Here's how the part is built. I have some questions about the finished solid (model axes, mm). A direction names the side the tool comes from. Coordinates: 2 decimals unless noted, no trailing zeros. Write each loop counter-clockwise with the first axis right and the second up, starting at its lowest first coordinate (ties: lowest second). Pieces come first, ordered by that corner, then holes.
(1) Imagine slicing it at A-A, the plane x = 0. List the corners of the cut face in (y, z) for me.
(2) Thinking about a two-plate mould opening in X: for faces 4 (the flat face through (-40, 0, 6)), 5 (the cylindrical face through (20.765, -39.923, -1.479)), 6 (the cylindrical face through (-3, 0, 0)), which applies, released by +X, released by -X, zero draft, split by the parting line, or undercut?
(3) Imagine slicing it at D-D, the plane x = -10. List the corners of the cut face in (y, z) for me, plus the area to 3 significant figures.
(4) Please list where these lines run through material, in increasing order: probe 1 along Y at (x, z) = (0, -2.5); probe 2 along Y at (x, z) = (18, 2); probe 3 along Y at (x, z) = (0, 1).
(5) Imagine slicing it at C-C, the plane z = 1.5. State how many separate pieces and enclosed holes the cut face has, plus the area to 3 significant figures.
(6) For pin 1 Ø5.5 at (x, y) = (0, 0) entering from -Z; pin 2 Ø4 at (x, y) = (-11.5, -0.5) entering from -Z; pin 3 Ø13 at (x, y) = (2, -1) entering from +Z; pin 4 Ø5 at (y, z) = (-34, -2) entering from +X, each with a flat end and sliding along its axis, tell me the tip position at first contact or that it passes through.
(7) Which directions (+Z, -Z, +X, -X, +Y, -Y) give clear straight access to the entire face, cutting with the end or side of a thin tool? Please do faces 1 (the flat face through (-3, -1, 4)), 2 (the flat face through (20, 0, 6)), 3 (the cylindrical face through (22.997, -34.773, 2.958)).
```python
from build123d import *

# Parameters (mm, degrees)
SKETCH_1_R           = 45
EXTRUDE_1_DEPTH      = 3
SKETCH_2_R           = 3
EXTRUDE_2_DEPTH      = 6
EXTRUDE_3_DEPTH      = 4
EXTRUDE_3_DEPTH_BACK = 5
SKETCH_3_R           = 6
CUT_EXTRUDE_1_REACH  = 66.273
SKETCH_4_R           = 3
SKETCH_5_R           = 3
EXTRUDE_4_DEPTH      = 6


with BuildPart() as part:
    # 草图1 → 凸台-拉伸1 (new body)
    with BuildSketch(Plane.XY):
        Circle(SKETCH_1_R)
    extrude(amount=-EXTRUDE_1_DEPTH)

    # 草图2 → 凸台-拉伸2 (add)
    with BuildSketch(Plane.XY):
        with Locations(Location((-40, 0, 0), (0, 0, 180))):
            Circle(SKETCH_2_R)
        with Locations(Location((-20, 34.641016151, 0), (0, 0, 180))):
            Circle(SKETCH_2_R)
        with Locations(Location((20, 34.641016151, 0), (0, 0, 180))):
            Circle(SKETCH_2_R)
        with Locations(Location((40, 0, 0), (0, 0, 180))):
            Circle(SKETCH_2_R)
        with Locations(Location((20, -34.641016151, 0), (0, 0, 180))):
            Circle(SKETCH_2_R)
        with Locations(Location((-20, -34.641016151, 0), (0, 0, 180))):
            Circle(SKETCH_2_R)
    extrude(amount=EXTRUDE_2_DEPTH)

    # 草图3 → 凸台-拉伸3 (add, two sides: drawn at the far end of the back side and taken through both)
    with BuildSketch(Plane.XY.offset(-EXTRUDE_3_DEPTH_BACK)):
        Circle(SKETCH_3_R)
    extrude(amount=EXTRUDE_3_DEPTH + EXTRUDE_3_DEPTH_BACK)

    # 草图4 → 切除-拉伸1 (cut, up to next)
    with BuildSketch(Plane.XY.offset(4), mode=Mode.PRIVATE) as cut_extrude_1_sk1:
        Circle(SKETCH_4_R)
    cut_extrude_1_tool1 = extrude(cut_extrude_1_sk1.sketch, amount=-CUT_EXTRUDE_1_REACH, mode=Mode.PRIVATE) & part.part
    add(cut_extrude_1_tool1.solids().sort_by_distance((0, 0, 4))[0], mode=Mode.SUBTRACT)

    # 草图5 → 凸台-拉伸4 (add)
    with BuildSketch(Plane.XY):
        with Locations((-20, 0)):
            Circle(SKETCH_5_R)
        with Locations((-10, 17.320508076)):
            Circle(SKETCH_5_R)
        with Locations((10, 17.320508076)):
            Circle(SKETCH_5_R)
        with Locations((20, 0)):
            Circle(SKETCH_5_R)
        with Locations((10, -17.320508076)):
            Circle(SKETCH_5_R)
        with Locations((-10, -17.320508076)):
            Circle(SKETCH_5_R)
    extrude(amount=EXTRUDE_4_DEPTH)


solid = part.part
```
Recorded:
1. outline: (-45, -3) - (-6, -3) - (-6, -5) - (-3, -5) - (-3, 4) - (-6, 4) - (-6, 0) - (-45, 0) - close; (3, -5) - (6, -5) - (6, -3) - (45, -3) - (45, 0) - (6, 0) - (6, 4) - (3, 4) - close
2. face 4: zero draft
2. face 5: split by the parting line
2. face 6: undercut
3. outline: (-43.87, -3) - (43.87, -3) - (43.87, 0) - (20.32, 0) - (20.32, 6) - (14.32, 6) - (14.32, 0) - (-14.32, 0) - (-14.32, 6) - (-20.32, 6) - (-20.32, 0) - (-43.87, 0) - close
3. area: 335 mm2
4. probe 1: y = -45 to -3, 3 to 45
4. probe 2: y = -36.88 to -32.4, -2.24 to 2.24, 32.4 to 36.88
4. probe 3: y = -6 to -3, 3 to 6
5. separate pieces: 13
5. enclosed holes: 1
5. area: 424 mm2
6. pin 1: passes through
6. pin 2: stops at z = -3
6. pin 3: stops at z = 4
6. pin 4: stops at x = 32.14
7. face 1: +Z, +Y, -Y
7. face 2: +Z, +X, -X, +Y, -Y
7. face 3: +Z
